Source: three-view drawing plus pictorial views. Frame: mm from the lowest corner of the part. A direction names the side the tool comes from. Coordinates: 2 decimals unless noted, no trailing zeros. Order: outer loops, then holes, each group sorted by start corner. A loop starts at its lowest first (then second) coordinate and runs counter-clockwise, first axis right, second up. Notation, with made-up numbers: M -38.75,40 L -3.75,40 A31 cw -3.75,70 Z; hole C 61,74 d5. An arc over 180 degrees is marked long. One line per question, with ' | ' between items.
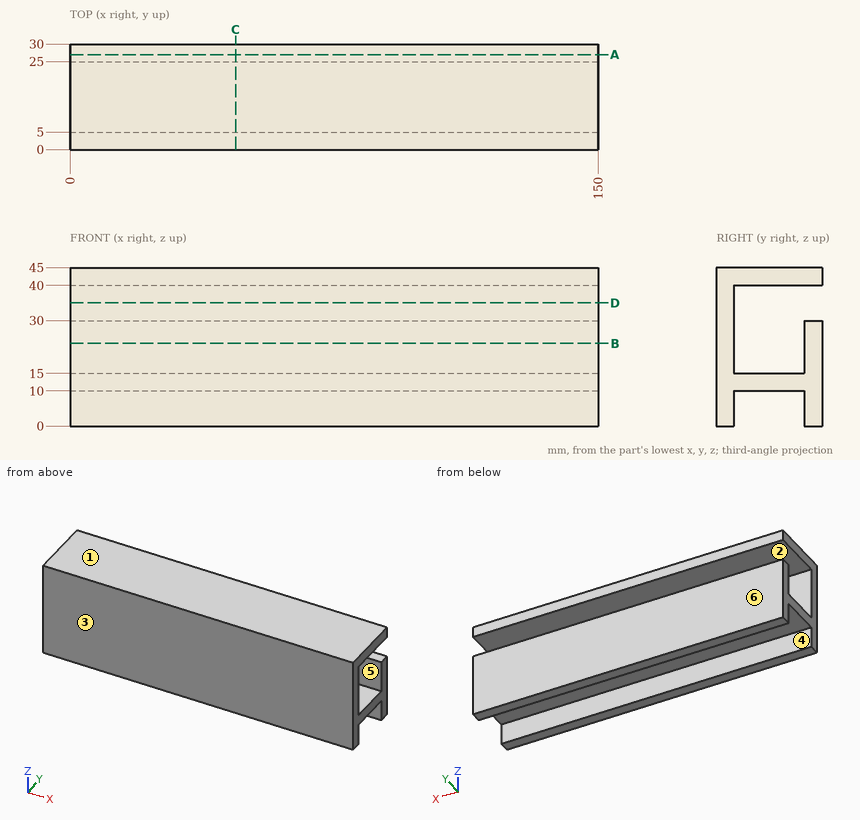
1. Section C-C, the plane x = 47. Output: boundary loops of the cut face in (y, z).
Response values:
outline: M 0,0 L 5,0 L 5,10 L 25,10 L 25,0 L 30,0 L 30,30 L 25,30 L 25,15 L 5,15 L 5,40 L 30,40 L 30,45 L 0,45 Z
2. Access query for the marked faces 4, 5 and 6. Directions: +Z, -Z, +X, -X, +Y, -Y. A direction counts if a zero-diameter tool reaches every point of the face in a straight line with its end or side. Return the directions, or none.
Response values:
face 4: -Z, +X, -X | face 5: +X, -X | face 6: +Z, -Z, +X, -X, +Y
3. Section D-D, the plane z = 35. Output: boundary loops of the cut face in (x, y).
Response values:
outline: M 0,0 L 150,0 L 150,5 L 0,5 Z
4. Draft query along Z for the marked faces 1, 2 and 3. Return one class per face: pulls with the +Z half, pulls with the -Z half, needs draft (parallel to the pull), parting line crosses it, or undercut.
Response values:
face 1: pulls with the +Z half | face 2: undercut | face 3: needs draft
5. Section B-B, the plane z = 23.5. Output: boundary loops of the cut face in (x, y), and give its area (3 significant figures).
Response values:
outline: M 0,0 L 150,0 L 150,5 L 0,5 Z; M 0,25 L 150,25 L 150,30 L 0,30 Z | area: 1,500 mm^2
6. Section A-A, the plane y = 27. Output: boundary loops of the cut face in (x, z), and give its area (3 significant figures).
Response values:
outline: M 0,0 L 150,0 L 150,30 L 0,30 Z; M 0,40 L 150,40 L 150,45 L 0,45 Z | area: 5,250 mm^2
7. Material intervals for line 1 (Z direction, x = 110, y = 6.25); line 2 (Z direction, x = 72, y = 28.75); line 3 (Y direction, x = 56, z = 25), sorted ascending. Write a range as [from, to].
Response values:
line 1: z = [10, 15], [40, 45] | line 2: z = [0, 30], [40, 45] | line 3: y = [0, 5], [25, 30]
8. Pin query (flat end, axial travel): P1, Ø10, axis at x = 62.5, y = 15.5, coming from the -Z side. Return the tip coordinate at first contact, or that it passes through.
Response values:
P1: stops at z = 10
